from build123d import *

# Parameters (mm, degrees)
BOSS_EXTRUDE1_DEPTH = 34
CUT_EXTRUDE1_DEPTH  = 30
SKETCH3_R           = 1.5
SKETCH3_R_2         = 5
CUT_EXTRUDE2_DEPTH  = 5
SKETCH4_W           = 22
SKETCH4_H           = 20
CUT_EXTRUDE3_DEPTH  = 6
SKETCH5_W           = 22
SKETCH5_H           = 20
CUT_EXTRUDE4_DEPTH  = 6
BOSS_EXTRUDE2_DEPTH = 10
SKETCH13_R          = 1.1
BOSS_EXTRUDE3_DEPTH = 10


with BuildPart() as part:
    # Sketch1 → Boss-Extrude1 (new body)
    with BuildSketch(Plane(origin=(0, 0, 0), x_dir=(1, 0, 0), z_dir=(0, 1, 0))):
        with BuildLine():
            Line((-76.081577676, -29.466634021), (-21.923666814, -14.650090384))
            ThreePointArc((-21.923666814, -14.650090384), (-19.017028504, -17.184879238), (-15.560151539, -18.894762991))
            Line((-15.560151539, -18.894762991), (-10.044056272, -74.622428409))
            ThreePointArc((-10.044056272, -74.622428409), (-50.159082361, -62.422374938), (-76.081577676, -29.466634021))
        make_face()
    extrude(amount=BOSS_EXTRUDE1_DEPTH)

    # Sketch2 → Cut-Extrude1 (cut)
    with BuildSketch(Plane.XZ):
        with BuildLine():
            Line((-15.616008473, 70.242360983), (-20.11040821, 23.685256516))
            ThreePointArc((-20.11040821, 23.685256516), (-22.281207254, 22.23411959), (-24.191874091, 20.454367051))
            Line((-24.191874091, 20.454367051), (-69.788119019, 33.047125828))
            ThreePointArc((-69.788119019, 33.047125828), (-47.337872486, 58.396456158), (-15.616008473, 70.242360983))
        make_face()
    extrude(amount=-CUT_EXTRUDE1_DEPTH, mode=Mode.SUBTRACT)

    # Sketch3 → Cut-Extrude2 (cut)
    with BuildSketch(Plane.XZ.offset(-30)):
        with Locations(Location((-26.678732616, 28.39195825, 0), (0, 0, 270))):
            Circle(SKETCH3_R)
        with Locations(Location((-53.760144922, 41.299208442, 0), (0, 0, 270))):
            Circle(SKETCH3_R)
        with Locations(Location((-29.04143221, 58.298774373, 0), (0, 0, 270))):
            Circle(SKETCH3_R)
        with Locations(Location((-39.804422608, 40.186637237, 0), (0, 0, 270))):
            Circle(SKETCH3_R_2)
    extrude(amount=-CUT_EXTRUDE2_DEPTH, mode=Mode.SUBTRACT)

    # Sketch4 → Cut-Extrude3 (cut)
    with BuildSketch(Plane(origin=(-22.190078988, 0, 2.142123878), x_dir=(0.09608851901557673, 0, 0.9953727927331515), z_dir=(-0.9953727927331515, 0, 0.09608851901557673))):
        with Locations((45.416815893, 10)):
            Rectangle(SKETCH4_W, SKETCH4_H)
    extrude(amount=-CUT_EXTRUDE3_DEPTH, mode=Mode.SUBTRACT)

    # Sketch5 → Cut-Extrude4 (cut)
    with BuildSketch(Plane(origin=(2.202244009, 0, 8.049713729), x_dir=(-0.9645546270217643, 0, 0.26388325352493547), z_dir=(-0.26388325352493547, 0, -0.9645546270217643))):
        with Locations((53.035036195, 10)):
            Rectangle(SKETCH5_W, SKETCH5_H)
    extrude(amount=-CUT_EXTRUDE4_DEPTH, mode=Mode.SUBTRACT)

    # Sketch10 → Boss-Extrude2 (add)
    with BuildSketch(Plane.XZ.offset(-30)):
        Polygon((-18.88301812, 36.399686031), (-16.769070701, 58.297887471), (-23.73668025, 58.970507104), (-25.850627669, 37.072305664), align=None)
        Polygon((-37.014944581, 23.995839242), (-58.221116276, 29.852554092), (-56.357621539, 36.599952655), (-35.151449843, 30.743237805), align=None)
    extrude(amount=BOSS_EXTRUDE2_DEPTH)

    # Sketch13 → Boss-Extrude3 (add)
    with BuildSketch(Plane.XZ.offset(-20)):
        with Locations(Location((-51.961198367, 29.679846926, 0), (0, 0, 90))):
            Circle(SKETCH13_R)
        with Locations(Location((-42.804014603, 27.150818354, 0), (0, 0, 90))):
            Circle(SKETCH13_R)
        with Locations(Location((-18.846348086, 52.390153669, 0), (0, 0, 90))):
            Circle(SKETCH13_R)
        with Locations(Location((-19.759189017, 42.934112138, 0), (0, 0, 90))):
            Circle(SKETCH13_R)
    extrude(amount=BOSS_EXTRUDE3_DEPTH)


solid = part.part
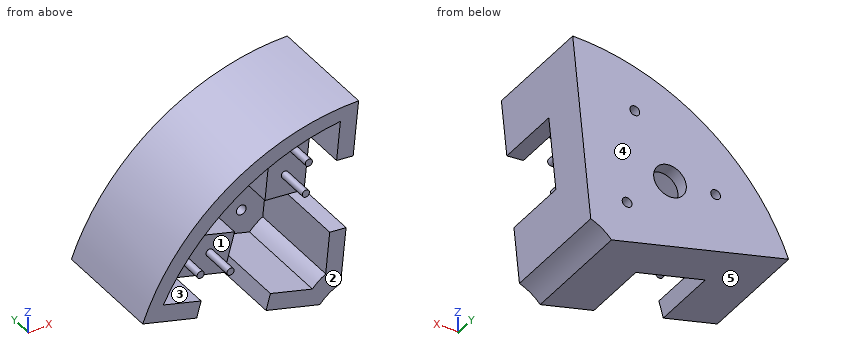
Input: part model. Units: mm. Frame: model coordinates. Face numbers are marked on the shaded views. A direction names the side the tool comes from. Coordinates: 2 decimals unless noted, no trailing zeros. Order: outer loops, then holes, each group sorted by start corner. A loop starts at its lowest first (then second) coordinate and runs counter-clockwise, first axis right, second up. Notation, with made-up numbers: M 58,54.25 L 69,54.25 A17 ccw 69,84.25 Z; hole C -31,59.5 d9. An arc over 180 degrees is marked long. Write item = value, one per line. Start each with the question number.
(1) Section B-B on y = 25.5. Output: boundary loops of the cut face in (x, z).
(2) Line query: line 1 along Y through (x, z) = (-19, 38.5); line 2 along Y through (x, z) = (-20, 35.5); line 3 along Z through (x, y) = (-53.5, 31.5). Output: solid intervals per line, ascending. Write a range as [from, to].
(3) First-contact query: P1, Ø0.7, axis at x = -43, z = 27, coming from the -Y side; P2, Ø3, axis at x = -56, y = 27, coming from the -Z side; P3, Ø3.5, axis at x = -26.68, z = 28.39, coming from the -Y side; P4, Ø2.5, axis at x = -53.76, z = 41.3, coming from the -Y side. Flat tips, straight axial feed; report the tip coordinate or a pass-through.
(4) Reachability of the marked faces 1 and 2 from +Z, -Z, +X, -X, +Y, -Y: full face, straight path, thin tool, end or side. Return the list, or none.
(5) Section D-D on z = 50.5. Output: boundary loops of the cut face in (x, y).
(6) Section A-A on y = 7. Output: boundary loops of the cut face in (x, z).
(7) Section C-C on x = -36. Output: boundary loops of the cut face in (y, z).
(8) Pull-direction query (X, two-part tool) for the marked faces 3, 4 and 5; classes: released by +X, released by -X, zero draft, split by the parting line, or undercut.
Result set:
q1.outline = M -76.08,29.47 L -21.92,14.65 A15 cw -15.56,18.89 L -10.04,74.62 A69.92 ccw Z; hole M -69.79,33.05 L -58.22,29.85 L -56.36,36.6 L -35.15,30.74 L -37.01,24 L -24.19,20.45 A16.27 cw -20.11,23.69 L -18.88,36.4 L -25.85,37.07 L -23.74,58.97 L -16.77,58.3 L -15.62,70.24 A70 ccw Z
q2.line_1 = [20, 34]
q2.line_2 = [30, 34]
q2.line_3 = [23.29, 39.82], [42.78, 59.99]
q3.P1 = 10
q3.P2 = 23.56
q3.P3 = 30
q3.P4 = through
q4.face_1 = -Y
q4.face_2 = +Z, -Z, +X, -X, -Y
q5.outline = M -63.53,0 L -56.9,0 L -56.9,30 L -24.55,30 L -24.55,20 L -12.43,20 L -12.43,34 L -63.53,34 Z
q6.outline = M -76.08,29.47 L -59.56,24.95 L -58.22,29.85 L -69.79,33.05 A70 cw -15.62,70.24 L -16.77,58.3 L -11.71,57.81 L -10.04,74.62 A69.92 ccw Z; M -38.34,19.14 L -21.92,14.65 A15 cw -15.56,18.89 L -13.88,35.92 L -18.88,36.4 L -20.11,23.69 A16.27 ccw -24.19,20.45 L -37.01,24 Z
q7.outline = M 0,18.5 L 34,18.5 L 34,36.94 L 30,36.94 L 30,30.98 L 20,30.98 L 20,27.67 L 30,27.67 L 30,23.72 L 0,23.72 Z; M 0,64.72 L 30,64.72 L 30,43.43 L 34,43.43 L 34,69.88 L 0,69.88 Z
q8.face_3 = undercut
q8.face_4 = zero draft
q8.face_5 = released by -X
